Can you work these out from the model? Positions are in its coordinate system, mm. A direction names the side the tool comes from. Coordinates: 2 decimals unless noted, no trailing zeros. Write each loop counter-clockwise with the first axis right and the second up, starting at its lowest first coordinate (ties: lowest second). Pieces come first, ordered by that corner, then holes.
```python
from build123d import *

# Parameters (mm, degrees)
ESQUISSE1_W        = 30
ESQUISSE1_H        = 30
BOSS_EXTRU_1_DEPTH = 15
ESQUISSE3_W        = 10
ESQUISSE3_H        = 15
BOSS_EXTRU_2_DEPTH = 5
CHANFREIN1_SIZE    = 30


with BuildPart() as part:
    # Esquisse1 → Boss.-Extru.1 (new body)
    with BuildSketch(Plane(origin=(0, 0, 0), x_dir=(1, 0, 0), z_dir=(0, 1, 0))):
        with Locations((15, -15)):
            Rectangle(ESQUISSE1_W, ESQUISSE1_H)
    extrude(amount=BOSS_EXTRU_1_DEPTH)

    # Esquisse3 → Boss.-Extru.2 (add)
    with BuildSketch(Plane(origin=(0, 0, 0), x_dir=(-1, 0, 0), z_dir=(0, 0, -1))):
        with Locations((-15, 7.5)):
            Rectangle(ESQUISSE3_W, ESQUISSE3_H)
    boss_extru_2 = extrude(amount=BOSS_EXTRU_2_DEPTH)

    # Symétrie1: Boss.-Extru.2 across plane
    add(boss_extru_2.mirror(Plane(origin=(0, 0, 0), x_dir=(0.7071067811865476, 0, 0.7071067811865475), z_dir=(0.7071067811865475, 0, -0.7071067811865476))))

    # Chanfrein1
    chanfrein1_edges = [part.edges().sort_by_distance(p)[0] for p in [
        (30, 7.5, 30),
    ]]
    chamfer(chanfrein1_edges, length=CHANFREIN1_SIZE - 0.0001)  # a hair under: the kernel refuses the full size


solid = part.part
```
1. I'm going to push flat-ended pins straight in: P1, Ø5.5, axis at x = -1.5, y = 8.5, coming from the -Z side; P2, Ø1.5, axis at y = 7.5, z = 25, coming from the +X side; P3, Ø3, axis at y = 6, z = 26, coming from the -X side. Where does each tip first touch, or does it pass through?
2. Which directions (+Z, -Z, +X, -X, +Y, -Y) give clear straight access to the entire face, cutting with the end or side of a thin tool? Please do faces 1 (the face through (-2, 7, 20)), 2 (the face through (5, 7, 0)), 3 (the face through (25, 7, 0)), 4 (the face through (15, 7, 15)).
3. If I drill on L1, parallel to X at y = 9.75, z = -1; L2, parallel to Z at x = 15.5, y = 13; L3, parallel to X at y = 1.75, z = 12.5, over which ranges is the centre line in solid material (lowest first)?
4. If we section it at C-C, the plane z = 15: List the corners of the cut face in (x, y) for me.
5. If we section it at B-B, the plane x = 22: List the corners of the cut face in (y, z) for me.
Answers:
1. P1: stops at z = 0
1. P2: stops at x = 5.75
1. P3: stops at x = 0
2. face 1: +Z, -X, +Y, -Y
2. face 2: -Z, -X, +Y, -Y
2. face 3: -Z, +X, +Y, -Y
2. face 4: +Z, +X, +Y, -Y
3. L1: x = 10 to 20
3. L2: z = -5 to 14.5
3. L3: x = -5 to 17.5
4. outline: (-5, 0) - (15, 0) - (15, 15) - (-5, 15) - close
5. outline: (0, 0) - (15, 0) - (15, 8) - (0, 8) - close
